The model under review builds one solid part; all positions refer to its coordinate system, in mm. A direction names the side the tool comes from. Give positions to 0.01 mm unless a question says otherwise; leave off trailing zeros. Order: outer loops, then holes, each group sorted by start corner. A loop starts at its lowest first (then second) coordinate and runs counter-clockwise, first axis right, second up. Notation, with made-up numbers: (-34, 25) -> (7, 25) arc R23 ccw to (7, 42) -> close; hole circle Ø5 at (-10, 64). An arc over 180 degrees is marked (long way). Use one line per item in the form item = value.
```python
from build123d import *

# Parameters (mm, degrees)
F1_DEPTH = 2
F2_W     = 30
F2_H     = 4
F3_DEPTH = 5
F4_R     = 1.15
F5_DEPTH = 25


with BuildPart() as f1:
    # F0 (on Front) → F1 (new body)
    with BuildSketch(Plane.XZ):
        Polygon((-32.254396, -12.737582), (-32.254396, -22.737582), (-32.254396, -32.737582), (30.745604, -32.737582), (30.745604, -12.737582), align=None)
    extrude(amount=F1_DEPTH)

    # F2 (on face) → F3 (join)
    with BuildSketch(Plane.XZ.offset(2)):
        with Locations((-8.754396, -25.737582)):
            Rectangle(F2_W, F2_H)
    extrude(amount=F3_DEPTH)

    # F4 (on face) → F5 (cut)
    with BuildSketch(Plane.XY.offset(-23.737582)):
        with Locations((-21.254396, -5)):
            Circle(F4_R)
        with Locations((3.745604, -5)):
            Circle(F4_R)
    extrude(amount=-F5_DEPTH, mode=Mode.SUBTRACT)


solid = f1.part
```
1. Add section B-B on z = -24.5. Give the boundary of the cut face in (x, y), then the cut area to 3 significant figures.
Values:
outline = (-32.25, -2) -> (-23.75, -2) -> (-23.75, -7) -> (6.25, -7) -> (6.25, -2) -> (30.75, -2) -> (30.75, 0) -> (-32.25, 0) -> close; hole circle Ø2.3 at (-21.25, -5); hole circle Ø2.3 at (3.75, -5)
area = 268 mm^2
2. For L1, parallel to Y at x = -28, z = -22.5; L2, parallel to Y at x = 4, z = -25.25; L3, parallel to X at y = -4.75, z = -25.5, list the stretches that pass through material, from the lowest coordinate up.
Values:
L1 = -2 to 0
L2 = -7 to -6.12, -3.88 to 0
L3 = -23.75 to -22.38, -20.13 to 2.62, 4.87 to 6.25
3. Add section D-D on z = -29. Give the boundary of the cut face in (x, y), then the cut area to 3 significant figures.
Values:
outline = (-32.25, -2) -> (30.75, -2) -> (30.75, 0) -> (-32.25, 0) -> close
area = 126 mm^2
4. Add section A-A on y = -5. Give the boundary of the cut face in (x, z).
Values:
outline = (-23.75, -27.74) -> (-22.4, -27.74) -> (-22.4, -23.74) -> (-23.75, -23.74) -> close; (-20.1, -27.74) -> (2.6, -27.74) -> (2.6, -23.74) -> (-20.1, -23.74) -> close; (4.9, -27.74) -> (6.25, -27.74) -> (6.25, -23.74) -> (4.9, -23.74) -> close
5. Add section C-C on x = -19.5. Give the boundary of the cut face in (y, z), then the cut area to 3 significant figures.
Values:
outline = (-7, -27.74) -> (-2, -27.74) -> (-2, -32.74) -> (0, -32.74) -> (0, -12.74) -> (-2, -12.74) -> (-2, -23.74) -> (-7, -23.74) -> close
area = 60.0 mm^2
6. The part is to be moulded in two halves that separate along Y. For faces 4 (the face through (-1, 0, -23)), 5 (the face through (-23.754, -4, -26)), 6 (the face through (4.36, -4.03, -25.71)), say which applies: +Y half, -Y half, draft (parallel to the pull), parting line (faces both ways), or undercut.
Values:
face_4 = +Y half
face_5 = draft
face_6 = undercut
7. Tool access review of faces 1 (the face through (6.246, -4, -26)), 2 (the face through (-9, -4, -27.738)), 3 (the face through (-9, -4, -23.738)): name each direction out of +Z, -Z, +X, -X, +Y, -Y from which nothing blocks a thin tool from reaching the whole face with its end or side.
Values:
face_1 = +Z, -Z, +X, -Y
face_2 = -Z, +X, -X, -Y
face_3 = +Z, +X, -X, -Y
8. For pin 1 Ø2 at (x, y) = (3.75, -5) entering from -Z (1 decimal); pin 2 Ø3 at (x, y) = (-21.25, -5) entering from +Z; pin 3 Ø4 at (x, y) = (-12.5, -5) entering from -Z; pin 4 Ø1.5 at (y, z) = (-6, -28) entering from +X, all flat-tipped, find the tip position at first contact; note any pin that passes through.
Values:
pin_1 = through
pin_2 = -23.74
pin_3 = -27.74
pin_4 = 6.25
